Study the drawing (mm; zero at the part's minimum x, y, z) and answer. A direction names the side the tool comes from. Give positions to 0.01 mm unless a question says otherwise; leave off trailing zeros. Write each loop counter-clockwise with the first axis right and the second up, starting at its lowest first coordinate (ties: lowest second). Pieces come first, ordered by that corner, then holes. Notation, with made-up numbers: (5, 39) - (41, 39) arc R20 ccw to (41, 64) - close; hole circle Ø8 at (-27.75, 26). An arc over 180 degrees is marked (long way). Return JSON: item names as keys, results as strings.
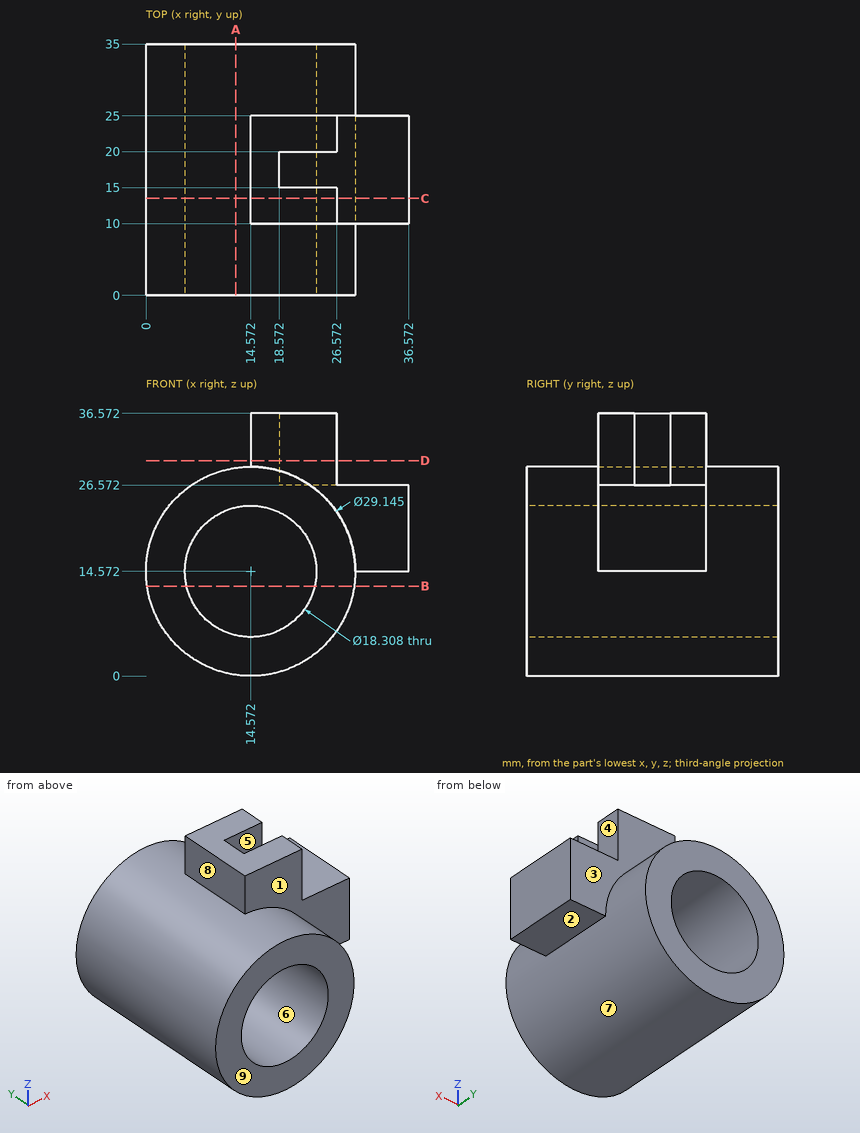
Item 1: Flat-ended cylindrical pins translate along their axes: P1, Ø2, axis at y = 21, z = 31, coming from the -X side; P2, Ø6, axis at y = 8, z = 6.5, coming from the -X side; P3, Ø1, axis at x = 4.5, y = 12.5, coming from the -Z side (1 decimal). Find the tip coordinate at first contact, or state that the pin passes through.
Answer below:
{"P1": "stops at x = 14.57", "P2": "stops at x = 0.91", "P3": "stops at z = 3.6"}
Item 2: For the marked faces 1, 2, 3, 4 and 5, determine the directions among +Z, -Z, +X, -X, +Y, -Y from which every point of the face is accessible in a straight line to the end or side of a thin tool.
Answer below:
{"face 1": "+Z, +X, -Y", "face 2": "-Z, +X, +Y, -Y", "face 3": "+Z, +X, +Y", "face 4": "+Z, +X, +Y, -Y", "face 5": "+Z, +X"}
Item 3: The mould has two halves that part along X. Classify the marked faces 6, 7, 8 and 9: +X half, -X half, draft (parallel to the pull), parting line (faces both ways), or undercut.
Answer below:
{"face 6": "undercut", "face 7": "parting line", "face 8": "-X half", "face 9": "draft"}
Item 4: A cutting plane is placed at D-D on z = 30. Determine the outline of the cut face in (x, y), then the cut area to 3 significant figures.
Answer below:
{"outline": "(14.57, 10) - (26.57, 10) - (26.57, 15) - (18.57, 15) - (18.57, 20) - (26.57, 20) - (26.57, 25) - (14.57, 25) - close", "area": "140 mm²"}
Item 5: A cutting plane is placed at C-C on y = 13.5. Determine the outline of the cut face in (x, z) (1 decimal).
Answer below:
{"outline": "(14.6, 29.1) arc R14.6 ccw (long way) to (29.1, 14.6) - (36.6, 14.6) - (36.6, 26.6) - (26.6, 26.6) - (26.6, 36.6) - (14.6, 36.6) - close; hole circle Ø18.3 at (14.6, 14.6)"}
Item 6: A cutting plane is placed at A-A on x = 12.5. Determine the outline of the cut face in (y, z).
Answer below:
{"outline": "(0, 0.15) - (35, 0.15) - (35, 5.66) - (0, 5.66) - close; (0, 23.49) - (35, 23.49) - (35, 29) - (0, 29) - close"}
Item 7: Consider L1, parallel to Z at x = 34, y = 23; L2, parallel to Y at x = 16.5, z = 33.5; L3, parallel to X at y = 17, z = 15.5 (1 decimal). Determine where each line is inside the solid, lowest interval first.
Answer below:
{"L1": "z = 14.57 to 26.57", "L2": "y = 10 to 25", "L3": "x = 0 to 5.5, 23.7 to 36.6"}
Item 8: A cutting plane is placed at B-B on z = 12.5. Determine the outline of the cut face in (x, y).
Answer below:
{"outline": "(0.15, 0) - (5.66, 0) - (5.66, 35) - (0.15, 35) - close; (23.49, 0) - (29, 0) - (29, 35) - (23.49, 35) - close"}
